Autodesk Inventor part; units mm, degrees
ref_plane "YZ Plane" through (0, 0, 0) normal (1, 0, 0) x (0, 1, 0)
ref_plane "XZ Plane" through (0, 0, 0) normal (0, 1, 0) x (-1, 0, 0)
ref_plane "XY Plane" through (0, 0, 0) normal (0, 0, 1) x (1, 0, 0)
sketch "Sketch1" plane through (0, 0, 0) normal (0, 1, 0) x (-1, 0, 0)
  line L0 (20, 45) -> (-20, 45)
  line L1 (-20, 45) -> (-20, -45)
  line L2 (-20, -45) -> (20, -45)
  line L3 (20, -45) -> (20, 45)
  line L4 (20, 45) -> (-20, -45) construction
  line L5 (-20, 45) -> (20, -45) construction
  line L6 (20, -45) -> (50, -45)
  line L7 (50, -45) -> (50, 45)
  line L8 (50, 45) -> (20, 45)
  line L9 (20, 45) -> (20, -45)
  point P0 (0, 0)
  dimension "d0" = 40
  dimension "d1" = 90
  dimension "d7" = 30
  dimension "d8" = 90
extrude "Extrusion1" add sketch "Sketch1" along normal blind 3.6
sketch "Sketch3" plane through (0, 3.6, 0) normal (0, 1, 0) x (1, 0, 0)
  line L0 (-50, 45) -> (-50, -45)
  circle A0 centre (-30, 45) radius 22.5
  point P0 (0, 0)
  point P1 (20, 45)
  dimension "d37" = 20
  dimension "d38" = 45
extrude "Extrusion3" cut sketch "Sketch3" against normal blind 10
fillet "Fillet2" radius 4 3 edges at (-50, 1.8, 45) (20, 1.8, 45) (-50, 1.8, -34.6922)
chamfer "Chamfer1" distance 20 angle 45 1 edges at (20, 1.8, -45)
fillet "Fillet4" radius 10 2 edges at (0, 1.8, -45) (20, 1.8, -25)
fillet "Fillet5" radius 5 1 edges at (-7.5, 1.8, -45)
sketch "Sketch9" plane through (0, 0, 0) normal (0, -1, 0) x (1, 0, 0)
  circle A0 centre (-46.5, 41.5) radius 1.5
  line L0 (-46, 45) -> (16, 45)
  line L1 (-50, -23.8754) -> (-50, 41)
  arc A1 (-50, -23.8754) -> (-43.5849, -27.064) centre (-46, -23.8754) ccw
  point P0 (0, 0)
  dimension "d70" = 3
  dimension "d72" = 3.5
  dimension "d73" = 3.5
extrude "Extrusion9" cut sketch "Sketch9" against normal blind 10
sketch "Sketch4" plane through (0, 3.6, 0) normal (0, 1, 0) x (1, 0, 0)
  circle A0 centre (-2, -20) radius 31
  line L0 (20, -41) -> (20, 45)
  line L1 (-46, -45) -> (16, -45)
  point P0 (0, 0)
  point P1 (20, 23.8754)
  dimension "d14" = 62
  dimension "d15" = 22
  dimension "d16" = 25
extrude "Extrusion4" add sketch "Sketch4" against normal blind 3.6
sketch "Sketch12" plane through (0, 3.6, 0) normal (0, 1, 0) x (1, 0, 0)
  arc A0 (19.8839, -41.9566) -> (20, 1.8403) centre (-2, -20) ccw
  circle A1 centre (-2, -20) radius 26.5
  point P0 (0, 0)
  dimension "d95" = 53
extrude "Extrusion12" cut sketch "Sketch12" against normal blind 10
fillet "Fillet8" radius 10 2 edges at (-20.3303, 1.8, 45) (20, 1.8, -1.8403)
sketch "Sketch7" plane through (-32.64, 0, 1.0706) normal (0, -1, 0) x (1, 0, 0)
  circle A0 centre (27.64, -42.5706) radius 1.5
  circle A1 centre (49.14, -22.5706) radius 1.5
  circle A2 centre (49.14, 40.4294) radius 1.5
  line L0 (25.8579, -46.0706) -> (23.6643, -46.0706)
  line L1 (52.64, 41) -> (52.64, -20.8579)
  line L2 (-20, -45) -> (-20, 41)
  line L3 (-16, 43.9294) -> (46, 43.9294)
  line L4 (-13.36, 43.9294) -> (48.64, 43.9294)
  line L5 (52.64, 39.9294) -> (52.64, -21.9285)
  point P0 (0, 0)
  dimension "d56" = 3
  dimension "d53" = 3
  dimension "d50" = 3
  dimension "d58" = 3.5
  dimension "d55" = 3.5
  dimension "d57" = 25
  dimension "d54" = 20
  dimension "d52" = 3.5
  dimension "d51" = 3.5
  dimension "d62" = 0
  dimension "d63" = 0
  dimension "d79" = 90
extrude "Extrusion7" cut sketch "Sketch7" against normal blind 10
sketch "Sketch13" plane through (0, 0, 0) normal (0, -1, 0) x (1, 0, 0)
  circle A0 centre (16.5, 41.5) radius 1.5
  arc A1 (19.9534, 34.8424) -> (9.4018, 43.9217) centre (16.5, 41.5) ccw
  circle A2 centre (-2, 20) radius 26.5
  circle A3 centre (-2, 20) radius 26.5
  circle A4 centre (16.5, 41.5) radius 2.7131
  point P0 (0, 0)
  dimension "d97" = 15
extrude "Extrusion13" add sketch "Sketch13" against normal blind 3.6 contours A2 A4 A1 | A2 A4 picked at (14.5458, 40.9715)
sketch "Sketch14" plane through (0, 0, 0) normal (0, -1, 0) x (1, 0, 0)
  arc A0 (-7.8959, -40.7978) -> (-43.5849, -27.064) centre (-30, -45) ccw
  line L0 (-13.2295, -30) -> (-50, 11.1246)
  line L1 (-50, -23.8754) -> (-50, 41)
  line L2 (-50, 11.1246) -> (-50, -45)
  line L3 (-50, -45) -> (-13.2295, -30)
  point P0 (0, 0)
  dimension "d100" = 35
  dimension "d101" = 15
extrude "Extrusion14" cut sketch "Sketch14" against normal blind 3.6
fillet "Fillet9" radius 5 1 edges at (-50, 1.8, 11.1246)
properties part number "p1"
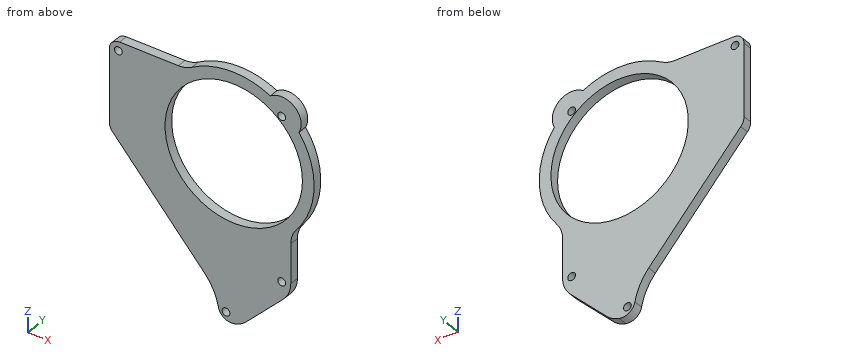
The listing builds one solid part. Answer for the finished solid, in the listing's coordinates (mm). Give positions to 0.01 mm unless a question says otherwise; leave off trailing zeros. Loops run counter-clockwise (first coordinate to the right, second up) from the corner with the lowest first, then second, coordinate; pieces in that order, holes last.
Item 1: A cutting plane is placed at C-C (y = 2.25). Give the vertices of the cut face in (x, z), then the cut area to 3 significant figures.
Derived:
outline: (-50, 13.03) arc R5 ccw to (-48.73, 9.7) - (-13.23, -30) arc R22.5 cw to (-7.9, -40.8) arc R5 ccw to (-1.83, -44.73) arc R10 ccw to (2.93, -42.07) - (17.07, -27.93) arc R10 ccw to (20, -20.86) - (20, -5.63) arc R10 cw to (22.2, 0.62) arc R31 ccw to (23.18, 38.09) arc R7.5 ccw to (12.13, 47.59) arc R31 ccw to (-18.15, 46.46) arc R10 cw to (-23.35, 45) - (-46, 45) arc R4 ccw to (-50, 41) - close; hole circle Ø3 at (-46.5, 41.5); hole circle Ø53 at (-2, 20); hole circle Ø3 at (-5, -41.5); hole circle Ø3 at (16.5, -21.5); hole circle Ø3 at (16.5, 41.5)
area: 2,960 mm2
Item 2: Find the intervals of material crossed by line 1 along Z through (x, y) = (16.5, 2.45); line 2 along X through (y, z) = (2.95, 19.5); line 3 along X through (y, z) = (3.15, 18), in increasing order.
Derived:
line 1: z = -28.5 to -23, -20 to 1.03, 38.97 to 40, 43 to 49
line 2: x = -50 to -28.5, 24.5 to 29
line 3: x = -50 to -28.42, 24.42 to 28.94
Item 3: A cutting plane is placed at D-D (x = -44). Give the vertices of the cut face in (y, z).
Derived:
outline: (0, 4.41) - (3.6, 4.41) - (3.6, 45) - (0, 45) - close
Item 4: A cutting plane is placed at B-B (x = -17). Give the vertices of the cut face in (y, z).
Derived:
outline: (0, -25.78) - (3.6, -25.78) - (3.6, -1.85) - (0, -1.85) - close; (0, 41.85) - (3.6, 41.85) - (3.6, 47.13) - (0, 47.13) - close
Item 5: A cutting plane is placed at A-A (z = 20). Give the vertices of the cut face in (x, y), then the cut area to 3 significant figures.
Derived:
outline: (-50, 0) - (-28.5, 0) - (-28.5, 3.6) - (-50, 3.6) - close; (24.5, 0) - (29, 0) - (29, 3.6) - (24.5, 3.6) - close
area: 93.6 mm2
Item 6: Each of these flat-tipped pins is pushed along its axis until it touches: pin 1 Ø2.5 at (x, z) = (-46.5, 41.5) entering from +Y; pin 2 Ø1 at (y, z) = (2, -27.5) entering from +X; pin 3 Ø1 at (x, y) = (-32.5, 1.5) entering from +Z. Where does it stop, or does it pass through?
Derived:
pin 1: passes through
pin 2: stops at x = 17.89
pin 3: stops at z = 45
